Answer from the drawing. Dimensions are ordinates in mm from the lowest x, y and z of the part. Coordinates: 2 decimals unless noted, no trailing zeros. Write each loop counter-clockwise with the first axis right and the second up, starting at its lowest first coordinate (ties: lowest second). Pieces come first, ordered by that corner, then holes. Notation, with made-up numbers: (43, -4.75) -> (55, -4.75) arc R27 ccw to (55, 24.25) -> close; hole circle Ø9 at (13, -3.75). An arc over 180 degrees is marked (long way). One line per item, written item: value. Start each with the question number.
1. Find section A-A, the plane y = 3.81. Write down the section's boundary in (x, z) (1 decimal).
2. Find section B-B, the plane x = 3.81. Write down the section's boundary in (y, z) (1 decimal).
3. For a pull along X with two mould halves and no side action, classify the marked faces 1, 2 and 3 as pulls with the +X half, pulls with the -X half, needs draft (parallel to the pull), parting line crosses it, or undercut.
4. Consider line 1 along Y through (x, z) = (3.81, 0.6); line 2 along X through (y, z) = (4.5, 3) (1 decimal); line 3 along X through (y, z) = (58.5, 1.25) (1 decimal). Determine where each line is inside the solid, lowest interval first.
5. Find section C-C, the plane z = 4. Write down the section's boundary in (x, y) (1 decimal), and give its area (3 significant figures).
6. Find section D-D, the plane x = 45. Write down the section's boundary in (y, z) (1 decimal).
7. Given P1, Ø3.5, axis at x = 96.266, y = 57.15, coming from the +Z side (1 decimal); P2, Ø2, axis at y = 4.5, z = 6, coming from the -X side; P3, Ø3.5, axis at x = 83.5, z = 5.5, coming from the +Y side, each flat-ended and moving along its own axis, determine where each tip first touches the part or whether it passes through.
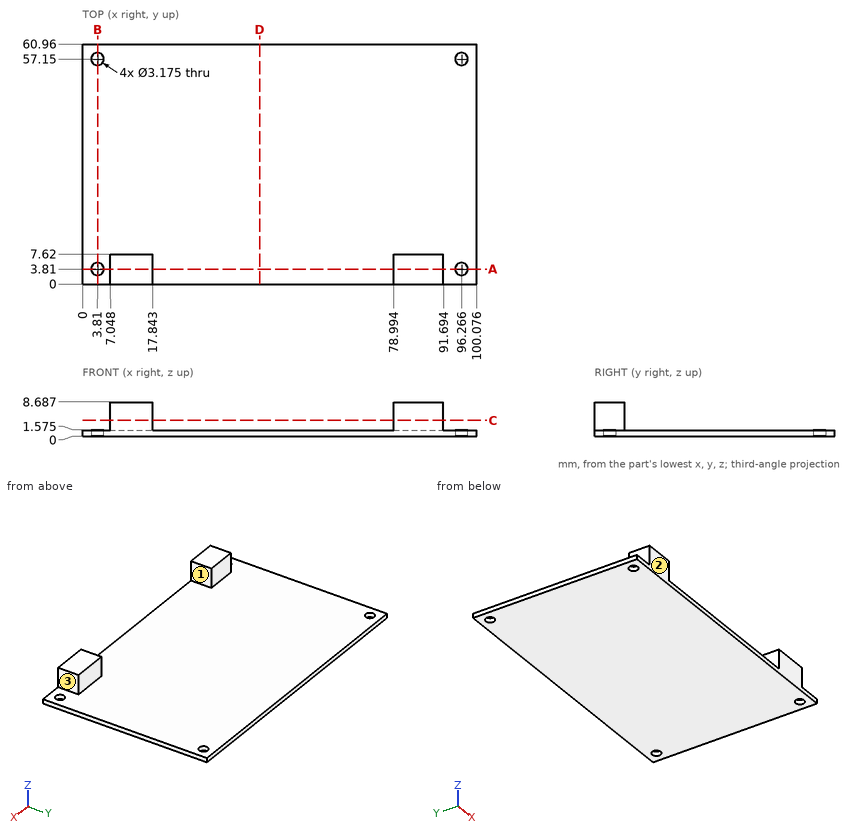
Answer block:
1. outline: (0, 0) -> (2.2, 0) -> (2.2, 1.6) -> (0, 1.6) -> close; (5.4, 0) -> (94.7, 0) -> (94.7, 1.6) -> (91.7, 1.6) -> (91.7, 8.7) -> (79, 8.7) -> (79, 1.6) -> (17.8, 1.6) -> (17.8, 8.7) -> (7, 8.7) -> (7, 1.6) -> (5.4, 1.6) -> close; (97.9, 0) -> (100.1, 0) -> (100.1, 1.6) -> (97.9, 1.6) -> close
2. outline: (0, 0) -> (2.2, 0) -> (2.2, 1.6) -> (0, 1.6) -> close; (5.4, 0) -> (55.6, 0) -> (55.6, 1.6) -> (5.4, 1.6) -> close; (58.7, 0) -> (61, 0) -> (61, 1.6) -> (58.7, 1.6) -> close
3. face 1: undercut
3. face 2: needs draft
3. face 3: pulls with the +X half
4. line 1: y = 0 to 2.22, 5.4 to 55.56, 58.74 to 60.96
4. line 2: x = 7 to 17.8, 79 to 91.7
4. line 3: x = 0 to 3, 4.6 to 95.4, 97.1 to 100.1
5. outline: (7, 0) -> (17.8, 0) -> (17.8, 7.6) -> (7, 7.6) -> close; (79, 0) -> (91.7, 0) -> (91.7, 7.6) -> (79, 7.6) -> close
5. area: 179 mm2
6. outline: (0, 0) -> (61, 0) -> (61, 1.6) -> (0, 1.6) -> close
7. P1: stops at z = 1.6
7. P2: stops at x = 7.05
7. P3: stops at y = 7.62
